from build123d import *

# Parameters (mm, degrees)
F0_W     = 63.5
F0_H     = 63.5
F1_DEPTH = 63.5
F2_R     = 14.2875
F3_DEPTH = 50.8
F2_R_2   = 25.4
F2_R_3   = 19.05
F4_DEPTH = 6.35
F5_W     = 46.99
F5_H     = 34.29
F6_DEPTH = 101.6
F7_SIZE  = 3.175
F8_R     = 3.175


with BuildPart() as f1:
    # F0 (on Top) → F1 (new body)
    with BuildSketch(Plane.XY):
        Rectangle(F0_W, F0_H)
    extrude(amount=F1_DEPTH)

    # F2 (on Top) → F3 (cut)
    with BuildSketch(Plane.XY):
        Circle(F2_R)
    extrude(amount=F3_DEPTH, mode=Mode.SUBTRACT)

    # F2 (on Top) → F4 (join)
    with BuildSketch(Plane.XY):
        Circle(F2_R_2)
        Circle(F2_R_3, mode=Mode.SUBTRACT)
    extrude(amount=-F4_DEPTH)

    # F5 (on Right) → F6 (join, symmetric)
    with BuildSketch(Plane.YZ):
        with Locations((0, 40.005002)):
            Rectangle(F5_W, F5_H)
    extrude(amount=F6_DEPTH, both=True)

    # F7
    f7_edges = [f1.edges().sort_by_distance(p)[0] for p in [
        (-31.75, -31.75, 31.75),
        (31.75, -31.75, 31.75),
        (0, -31.75, 0),
        (0, -31.75, 63.5),
        (31.75, 0, 63.5),
        (31.75, 0, 0),
        (-31.75, 0, 63.5),
        (0, 31.75, 63.5),
        (-31.75, 0, 0),
        (0, 31.75, 0),
        (-31.75, 31.75, 31.75),
        (31.75, 31.75, 31.75),
    ]]
    chamfer(f7_edges, length=F7_SIZE)

    # F8
    f8_edges = [f1.edges().sort_by_distance(p)[0] for p in [
        (66.675, -23.495, 57.150002),
        (-66.675, -23.495, 57.150002),
        (66.675, 23.495, 57.150002),
        (-66.675, 23.495, 57.150002),
        (-101.6, 0, 57.150002),
        (-101.6, 0, 22.860002),
        (-101.6, -23.495, 40.005002),
        (-101.6, 23.495, 40.005002),
        (66.675, -23.495, 22.860002),
        (-66.675, -23.495, 22.860002),
        (66.675, 23.495, 22.860002),
        (-66.675, 23.495, 22.860002),
        (101.6, 23.495, 40.005002),
        (101.6, 0, 57.150002),
        (101.6, 0, 22.860002),
        (101.6, -23.495, 40.005002),
    ]]
    fillet(f8_edges, radius=F8_R)


solid = f1.part
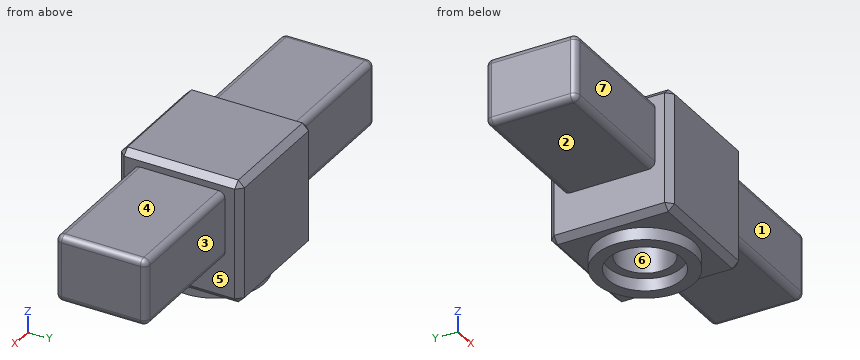
The model under review builds one solid part; all positions refer to its coordinate system, in mm. Face numbers are marked on the shaded views. A direction names the side the tool comes from. Coordinates: 2 decimals unless noted, no trailing zeros. Loops run counter-clockwise (first coordinate to the right, second up) from the corner with the lowest first, then second, coordinate; pieces in that order, holes last. Notation, with made-up numbers: M 87.5,21.5 L 95.5,21.5 A26 ccw 95.5,56.5 Z; hole C 19,1.25 d1. An arc over 180 degrees is marked long. Put each result on its own line as item: value. Start each with the question number.
Q1. Add section D-D (z = 40). Write out the cut boundary in (x, y) (3 decimals).
Q2. Wall thickness on line 1 (X direction, y = 0, z = 14.25); line 2 (Y direction, x = 0, z = -2.25): over which ranges is each line inside the solid? List them lowest first.
Q3. Clearance check with flat-ended pins moving along their axes: pin 1 (20.5 mm diameter, centred on x = 68.5, y = -5.5, fed in from -Z); pin 2 (12 mm diameter, centred on y = 3.5, z = 23, fed in from -X); pin 3 (5 mm diameter, centred on x = -74.5, z = 32.5, fed in from -Y) (3 decimals); pin 4 (3 mm diameter, centred on y = 24, z = 4.5, fed in from +X). State where each tip first meets the part, or that it passes through.
Q4. Add section B-B (x = -38). Write out the cut boundary in (y, z) (3 decimals), and give its area (3 significant figures).
Q5. The part is to be moulded in two halves that separate along Y. For the marked faces 5, 6 and 7, say which applies: +Y half, -Y half, draft (parallel to the pull), parting line (faces both ways), or undercut.
Q6. For the marked faces 1, 2, 3 and 4, list the 3-axis set-ups (+Z, -Z, +X, -X, +Y, -Y) from which the entire face can be reached by the end or side of a thin tool; tool diameter is ignored.
Answers:
1. outline: M -101.6,-20.32 A3.175 ccw -98.425,-23.495 L -31.75,-23.495 L -31.75,-28.575 L -28.575,-31.75 L 28.575,-31.75 L 31.75,-28.575 L 31.75,-23.495 L 98.425,-23.495 A3.175 ccw 101.6,-20.32 L 101.6,20.32 A3.175 ccw 98.425,23.495 L 31.75,23.495 L 31.75,28.575 L 28.575,31.75 L -28.575,31.75 L -31.75,28.575 L -31.75,23.495 L -98.425,23.495 A3.175 ccw -101.6,20.32 Z
2. line 1: x = -31.75 to -14.29, 14.29 to 31.75
2. line 2: y = -25.4 to -19.05, 19.05 to 25.4
3. pin 1: stops at z = 22.86
3. pin 2: stops at x = -101.6
3. pin 3: stops at y = -23.495
3. pin 4: stops at x = 31.75
4. outline: M -23.495,26.035 A3.175 ccw -20.32,22.86 L 20.32,22.86 A3.175 ccw 23.495,26.035 L 23.495,53.975 A3.175 ccw 20.32,57.15 L -20.32,57.15 A3.175 ccw -23.495,53.975 Z
4. area: 1,600 mm^2
5. face 5: draft
5. face 6: undercut
5. face 7: -Y half
6. face 1: +Z, -Z, +X, -Y
6. face 2: -Z, -X, +Y, -Y
6. face 3: +Z, -Z, +X, +Y
6. face 4: +Z, +X, +Y, -Y
